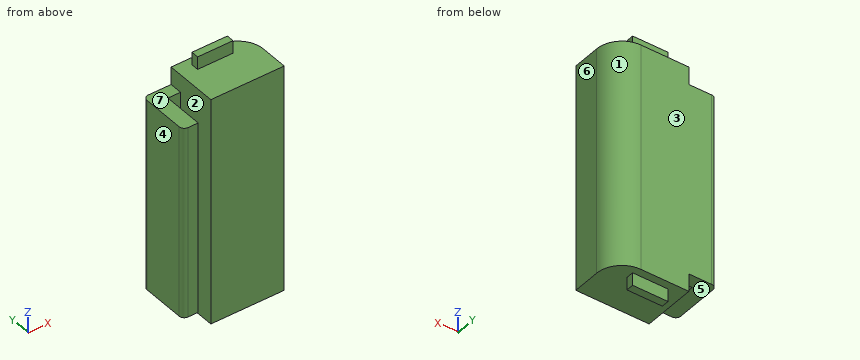
from build123d import *

# Parameters (mm, degrees)
BOSS_EXTRUDE1_DEPTH = 96.52
SKETCH3_W           = 36.83
SKETCH3_H           = 26.67
BOSS_EXTRUDE3_DEPTH = 8.89
SKETCH2_W           = 17.78
SKETCH2_H           = 3.81
BOSS_EXTRUDE4_DEPTH = 6.35
FILLET1_R           = 12.7
FILLET2_R           = 2.54


with BuildPart() as part:
    # Sketch1 → Boss-Extrude1 (new body)
    with BuildSketch(Plane.XY):
        Polygon((0, 0), (0, -20.32), (-7.62, -20.32), (-7.62, 6.35), (43.18, 6.35), (43.18, -20.32), (6.35, -20.32), (6.35, 0), align=None)
    extrude(amount=BOSS_EXTRUDE1_DEPTH)

    # Sketch3 → Boss-Extrude3 (add)
    with BuildSketch(Plane.XY.offset(96.52)):
        with Locations((24.765, -6.985)):
            Rectangle(SKETCH3_W, SKETCH3_H)
    boss_extrude3 = extrude(amount=BOSS_EXTRUDE3_DEPTH)

    # Sketch2 → Boss-Extrude4 (add)
    with BuildSketch(Plane(origin=(0, 0, 105.41), x_dir=(-1, 0, 0), z_dir=(0, 0, -1))):
        with Locations((-22.86, 0.635)):
            Rectangle(SKETCH2_W, SKETCH2_H)
    boss_extrude4 = extrude(amount=-BOSS_EXTRUDE4_DEPTH)

    # Mirror2: Boss-Extrude3, Boss-Extrude4 across plane
    add(boss_extrude3.mirror(Plane(origin=(0, 0, 48.26), x_dir=(1, 0, 0), z_dir=(0, 0, -1))))
    add(boss_extrude4.mirror(Plane(origin=(0, 0, 48.26), x_dir=(1, 0, 0), z_dir=(0, 0, -1))))

    # Fillet1
    fillet1_edges = [part.edges().sort_by_distance(p)[0] for p in [
        (43.18, 6.35, 48.26),
    ]]
    fillet(fillet1_edges, radius=FILLET1_R)

    # Fillet2
    fillet2_edges = [part.edges().sort_by_distance(p)[0] for p in [
        (-7.62, -20.32, 48.26),
        (-7.62, 6.35, 48.26),
    ]]
    fillet(fillet2_edges, radius=FILLET2_R)


solid = part.part
Input: part model. Units: mm. Frame: model coordinates. Face numbers are marked on the shaded views. A direction names the side the tool comes from. Give positions to 0.01 mm unless a question says otherwise; leave off trailing zeros. Write each loop counter-clockwise with the first axis right and the second up, starting at its lowest first coordinate (ties: lowest second). Pieces come first, ordered by that corner, then holes. Notation, with made-up numbers: M -26,43.5 L 6,43.5 A28 cw 6,78.5 Z; hole C 64.25,84.5 d11. An arc over 180 degrees is marked long. Use one line per item in the form item = value.
1. Cut plane B-B on z = 26. Return loops of the section in (x, y), and give its area (3 significant figures).
Outcome:
outline = M -7.62,-17.78 A2.54 ccw -5.08,-20.32 L 0,-20.32 L 0,0 L 6.35,0 L 6.35,-20.32 L 43.18,-20.32 L 43.18,-6.35 A12.7 ccw 30.48,6.35 L -5.08,6.35 A2.54 ccw -7.62,3.81 Z
area = 1,190 mm²
2. Cut plane D-D on x = 12.5. Return loops of the section in (y, z).
Outcome:
outline = M -20.32,-8.89 L 6.35,-8.89 L 6.35,105.41 L -20.32,105.41 Z
3. Mould query, pull axis X, two halves, no side actions, for the marked faces 1, 2, 3 and 4. Classes: released by +X, released by -X, zero draft, split by the parting line, or undercut.
Outcome:
face_1 = released by +X
face_2 = undercut
face_3 = zero draft
face_4 = released by -X
4. Cut plane C-C on x = 22. Return loops of the section in (y, z), and give its area (3 significant figures).
Outcome:
outline = M -20.32,-8.89 L -1.27,-8.89 L -1.27,-15.24 L 2.54,-15.24 L 2.54,-8.89 L 6.35,-8.89 L 6.35,105.41 L 2.54,105.41 L 2.54,111.76 L -1.27,111.76 L -1.27,105.41 L -20.32,105.41 Z
area = 3,100 mm²
5. Reachability of the marked faces 5, 6 and 7 from +Z, -Z, +X, -X, +Y, -Y: full face, straight path, thin tool, end or side. Return the list, or none.
Outcome:
face_5 = -Z, -X, +Y, -Y
face_6 = +Z, -Z, +X, +Y, -Y
face_7 = +Z, -X, +Y, -Y
6. Cut plane A-A on y = -8.5. Return loops of the section in (x, z), and give its area (3 significant figures).
Outcome:
outline = M -7.62,0 L 0,0 L 0,96.52 L -7.62,96.52 Z; M 6.35,-8.89 L 43.18,-8.89 L 43.18,105.41 L 6.35,105.41 Z
area = 4,950 mm²
7. Ray query, L1, parallel to X at y = -12.5, z = 9.5; L2, parallel to X at y = -3.75, z = 40.5; L3, parallel to Z at x = 7, y = -16.75. Return the intervals inside material, ascending.
Outcome:
L1 = -7.62 to 0, 6.35 to 43.18
L2 = -7.62 to 0, 6.35 to 42.91
L3 = -8.89 to 105.41
8. First-contact query: P1, Ø11, axis at x = 1.5, y = -2, coming from the -Z side; P2, Ø15.5, axis at x = 1.5, y = -13, coming from the +Z side; P3, Ø1.9, axis at y = 1, z = -13.5, coming from the -X side. Flat tips, straight axial feed; report the tip coordinate or a pass-through.
Outcome:
P1 = -8.89
P2 = 105.41
P3 = 13.97
